Could you check a few things on this model? Use its own coordinates, in mm. A direction names the side the tool comes from. Give positions to 0.01 mm unless a question says otherwise; leave off trailing zeros. Loops run counter-clockwise (first coordinate to the right, second up) from the corner with the lowest first, then second, coordinate; pieces in that order, holes last. Notation, with made-up numbers: (37.25, -25.5) -> (54.25, -25.5) arc R23 cw to (54.25, 9.5) -> close; hole circle Ø8 at (33.25, 67). An arc over 180 degrees is marked (long way). Write item = value, one per line. Start each with the question number.
1) I want a section at C-C (z = 15.5). List the corners of the cut face in (x, y) for me.
2) I need wall thicknesses on probe 1 along X at (y, z) = (2, 60); probe 2 along X at (y, z) = (3.7, 29); probe 3 along X at (y, z) = (1.3, 20.5). Which ranges of each line are inside material? Lowest first, please. Write a range as from..to.
3) If we mould it in two halves opening along X, with no side actions, what happens to faces 3 (the face through (62.785, 2.465, 41.899)), 4 (the face through (140, 2, -45)), 5 (the face through (-140, 2, -1))? For each: +X half, -X half, draft (parallel to the pull), parting line (faces both ways), or undercut.
4) I want a section at A-A (x = -94.5). List the corners of the cut face in (y, z) for me, and give its area (3 significant figures).
5) I'm going to push flat-ended pins straight in: pin 1 Ø12 at (x, z) = (80.5, 47.5) entering from -Y; pin 2 Ø2.5 at (x, y) = (128.5, 2) entering from +Z. Where does each tip first touch, or does it pass through?
6) On a 3-axis mill with a long thin cutter (end or side, diameter ignored), from which of +Z, -Z, +X, -X, +Y, -Y can I reach the whole of each face in a straight line? I mean faces 1 (the face through (-2, 5, -1)), 2 (the face through (120, 2, 36)). Say none if no direction works.
7) I want a section at B-B (y = 3.85). Count the separate pieces of the cut face and the enclosed holes in it, and give its area (3 significant figures).
from build123d import *

# Parameters (mm, degrees)
SKETCH_1_R      = 1.6
SKETCH_1_R_2    = 12
SKETCH_1_R_3    = 2.1
SKETCH_1_R_4    = 2.2
EXTRUDE_1_DEPTH = 5


with BuildPart() as part:
    # 草图1 → 凸台-拉伸1 (new body)
    with BuildSketch(Plane(origin=(0, 0, 0), x_dir=(1, 0, 0), z_dir=(0, 1, 0))):
        Polygon((-140, 80), (-140, -80), (120, -80), (120, 10), (140, 10), (140, 80), align=None)
        with Locations(Location((-110, -60, 0), (0, 0, 270))):
            Circle(SKETCH_1_R, mode=Mode.SUBTRACT)
        with Locations(Location((-79, -60, 0), (0, 0, 270))):
            Circle(SKETCH_1_R, mode=Mode.SUBTRACT)
        with Locations(Location((-94.5, -44.5, 0), (0, 0, 270))):
            Circle(SKETCH_1_R_2, mode=Mode.SUBTRACT)
        with Locations(Location((-65, -45.5, 0), (0, 0, 270))):
            Circle(SKETCH_1_R_3, mode=Mode.SUBTRACT)
        with Locations(Location((-110, -29, 0), (0, 0, 270))):
            Circle(SKETCH_1_R, mode=Mode.SUBTRACT)
        with Locations(Location((-79, -29, 0), (0, 0, 270))):
            Circle(SKETCH_1_R, mode=Mode.SUBTRACT)
        with Locations(Location((-65, -20.5, 0), (0, 0, 270))):
            Circle(SKETCH_1_R_3, mode=Mode.SUBTRACT)
        with Locations(Location((59, -60, 0), (0, 0, 270))):
            Circle(SKETCH_1_R_4, mode=Mode.SUBTRACT)
        with Locations(Location((45, -45.5, 0), (0, 0, 270))):
            Circle(SKETCH_1_R_3, mode=Mode.SUBTRACT)
        with Locations(Location((90, -60, 0), (0, 0, 270))):
            Circle(SKETCH_1_R_4, mode=Mode.SUBTRACT)
        with Locations(Location((74.5, -44.5, 0), (0, 0, 270))):
            Circle(SKETCH_1_R_2, mode=Mode.SUBTRACT)
        with Locations(Location((45, -20.5, 0), (0, 0, 270))):
            Circle(SKETCH_1_R_3, mode=Mode.SUBTRACT)
        with Locations(Location((59, -29, 0), (0, 0, 270))):
            Circle(SKETCH_1_R_4, mode=Mode.SUBTRACT)
        with Locations(Location((90, -29, 0), (0, 0, 270))):
            Circle(SKETCH_1_R, mode=Mode.SUBTRACT)
        with Locations(Location((87, 0, 0), (0, 0, 270))):
            Circle(SKETCH_1_R, mode=Mode.SUBTRACT)
        with Locations(Location((72, 70, 0), (0, 0, 270))):
            Circle(SKETCH_1_R, mode=Mode.SUBTRACT)
        with Locations(Location((135, 70, 0), (0, 0, 270))):
            Circle(SKETCH_1_R, mode=Mode.SUBTRACT)
    extrude(amount=EXTRUDE_1_DEPTH)


solid = part.part
Answer list:
q1.outline = (-140, 0) -> (120, 0) -> (120, 5) -> (-140, 5) -> close
q2.probe_1 = -140..-111.6, -108.4..-80.6, -77.4..56.8, 61.2..87.8, 92.2..120
q2.probe_2 = -140..-111.6, -108.4..-80.6, -77.4..56.8, 61.2..88.4, 91.6..120
q2.probe_3 = -140..-67.1, -62.9..42.9, 47.1..120
q3.face_3 = undercut
q3.face_4 = +X half
q3.face_5 = -X half
q4.outline = (0, -80) -> (5, -80) -> (5, 32.5) -> (0, 32.5) -> close; (0, 56.5) -> (5, 56.5) -> (5, 80) -> (0, 80) -> close
q4.area = 680 mm^2
q5.pin_1 = 0
q5.pin_2 = -10
q6.face_1 = +Z, -Z, +X, -X, +Y
q6.face_2 = +Z, +X, +Y, -Y
q7.separate_pieces = 1
q7.enclosed_holes = 17
q7.area = 41,900 mm^2
